from build123d import *

# Parameters (mm, degrees)
SKETCH_1_R            = 2.35
EXTRUDE_248_DEPTH     = 2.5
CUT_EXTRUDE_382_DEPTH = 1.1
SKETCH_3_R            = 1.25
EXTRUDE_487_DEPTH     = 100


with BuildPart() as part:
    # 草图1 → Extrude 248 (new body)
    with BuildSketch(Plane(origin=(0, 0, 0), x_dir=(1, 0, 0), z_dir=(0, 1, 0))):
        Circle(SKETCH_1_R)
    extrude(amount=EXTRUDE_248_DEPTH)

    # 草图2 → Cut-Extrude 382 (cut)
    with BuildSketch(Plane(origin=(0, 2.5, 0), x_dir=(1, 0, 0), z_dir=(0, 1, 0))):
        Polygon((1.154700538, 0), (0.577350269, 1), (-0.577350269, 1), (-1.154700538, 0), (-0.577350269, -1), (0.577350269, -1), align=None)
    extrude(amount=-CUT_EXTRUDE_382_DEPTH, mode=Mode.SUBTRACT)

    # 草图3 → Extrude 487 (add)
    with BuildSketch(Plane.XZ):
        Circle(SKETCH_3_R)
    extrude(amount=EXTRUDE_487_DEPTH)


solid = part.part
Work out the finished part from the listing and answer in its coordinate system (mm). A direction names the side the tool comes from. Give positions to 0.01 mm unless a question says otherwise; leave off trailing zeros. Loops run counter-clockwise (first coordinate to the right, second up) from the corner with the lowest first, then second, coordinate; pieces in that order, holes last. Notation, with made-up numbers: (17, -18) - (72, -18) arc R22 ccw to (72, -2) - close; hole circle Ø5 at (57.25, 3). An arc over 180 degrees is marked (long way). Answer in a Markdown table with one row per item. Add a question column.
Q1. Determine the mould class of faces 1 (the flat face through (1, 0, 1)), 2 (the flat face through (0, 1.4, 0)), 3 (the cylindrical face through (-0.509, 1.232, 2.294)) for opening direction Z: released by +Z, released by -Z, zero draft, split by the parting line, or undercut.
Q2. Each of these flat-tipped pins is pushed along its axis until it touches: P1, Ø1, axis at x = 1, y = -37, coming from the -Z side; P2, Ø1, axis at y = -69.5, z = -0.5, coming from the -X side; P3, Ø2, axis at x = -1, y = -85, coming from the +Z side. Where does it stop, or does it pass through?
Q3. The part is cut by section A-A (y = -39). Determine the outline of the cut face in (x, z), and give its area (3 significant figures).
Q4. A tool of negligible diameter and unlimited length cuts with its end or side. For faces 4 (the flat face through (0, -100, 0)), 5 (the cylindrical face through (-0.27, -49.3, -1.22)), from which of +Z, -Z, +X, -X, +Y, -Y can it reach the whole face along a straight path? Write none if from no direction.
Q5. Consider line 1 along Y through (x, z) = (-0.9, -2.05); line 2 along Z through (x, y) = (-0.15, -15); line 3 along Y through (x, z) = (0.55, 0.1). Determine where each line is inside the solid, lowest interval first.
Solution:
| question | item | result |
|---|---|---|
| 1 | face 1 | zero draft |
| 1 | face 2 | undercut |
| 1 | face 3 | split by the parting line |
| 2 | P1 | stops at z = -1.15 |
| 2 | P2 | stops at x = -1.25 |
| 2 | P3 | stops at z = 1.25 |
| 3 | outline | circle Ø2.5 at (0, 0) |
| 3 | area | 4.91 mm² |
| 4 | face 4 | +Z, -Z, +X, -X, -Y |
| 4 | face 5 | -Y |
| 5 | line 1 | y = 0 to 2.5 |
| 5 | line 2 | z = -1.24 to 1.24 |
| 5 | line 3 | y = -100 to 1.4 |
